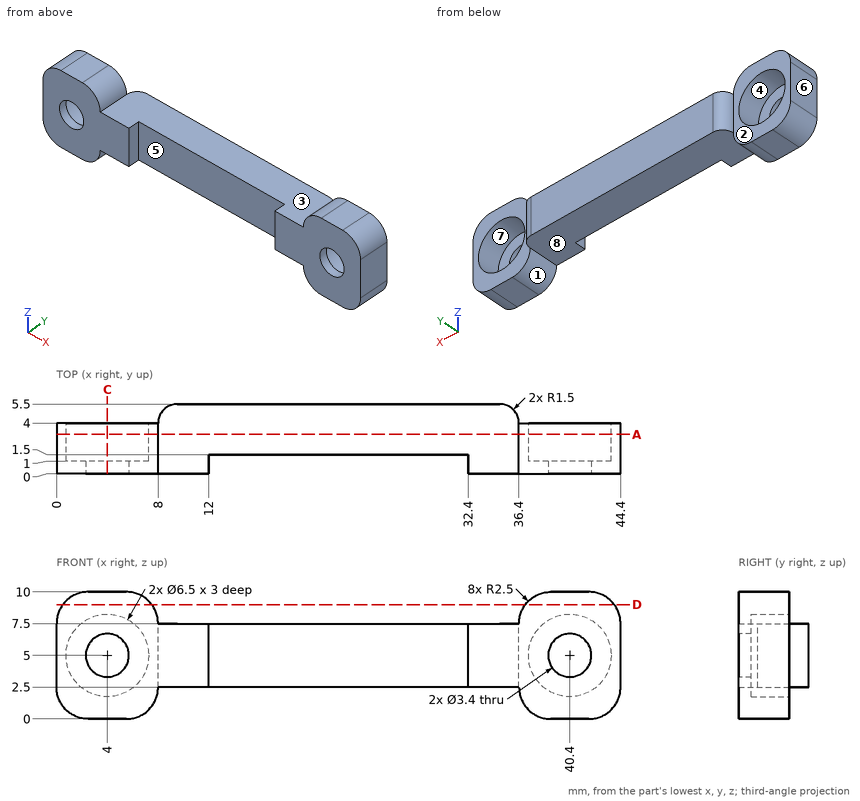
Job drawing, mm, ordinate dimensions from the low corner. One solid piece. A direction names the side the tool comes from. Give positions to 0.01 mm unless a question says otherwise; leave off trailing zeros. Order: outer loops, then holes, each group sorted by start corner. A loop starts at its lowest first (then second) coordinate and runs counter-clockwise, first axis right, second up. Notation, with made-up numbers: (-22, -26.75) -> (-11, -26.75) arc R31 cw to (-11, 5.25) -> close; hole circle Ø5 at (-33.5, 15). An arc over 180 degrees is marked (long way). Return JSON: item names as keys, results as strings.
Q1. Saw through at C-C (x = 4). Write the cut outline in (y, z), then the cut area to 3 significant figures.
Working result:
{"outline": "(0, 0) -> (4, 0) -> (4, 1.75) -> (1, 1.75) -> (1, 3.3) -> (0, 3.3) -> close; (0, 6.7) -> (1, 6.7) -> (1, 8.25) -> (4, 8.25) -> (4, 10) -> (0, 10) -> close", "area": "17.1 mm²"}
Q2. Saw through at A-A (y = 3.1). Count the separate pieces of the cut face and the enclosed holes in it, then the cut area to 3 significant figures.
Working result:
{"separate pieces": "1", "enclosed holes": "2", "area": "225 mm²"}
Q3. Mould opens along Z. For the marked faces 6, 7 and 8 say: pulls with the +Z half, pulls with the -Z half, needs draft (parallel to the pull), parting line crosses it, or undercut.
Working result:
{"face 6": "needs draft", "face 7": "undercut", "face 8": "pulls with the -Z half"}
Q4. Which spindle directions (+Z, -Z, +X, -X, +Y, -Y) get a long thin tool onto all of the face, cutting with end or side? Do the marked faces 1, 2, 3, 4 and 5. Say none if no direction does.
Working result:
{"face 1": "-Z, +Y, -Y", "face 2": "+Z, -Z, -X, +Y", "face 3": "+Z, +Y, -Y", "face 4": "+Y", "face 5": "+Z, -Z, -Y"}
Q5. Drill centre lines: line 1 (X direction, y = 0.75, z = 5); line 2 (X direction, y = 1.7, z = 4.75); line 3 (Z direction, x = 4, y = 2.05). Where is each one in solid material? Low to high.
Working result:
{"line 1": "0 to 2.3, 5.7 to 12, 32.4 to 38.7, 42.1 to 44.4", "line 2": "0 to 0.76, 7.24 to 37.16, 43.64 to 44.4", "line 3": "0 to 1.75, 8.25 to 10"}
Q6. Flat gauge pins, fed straight in: pin 1 (2.5 mm diameter, centred on x = 39.5, z = 6.5, fed in from +Y); pin 2 (1.5 mm diameter, centred on x = 34.5, y = 2, fed in from +Z); pin 3 (3 mm diameter, centred on x = 29, y = 4, fed in from -Z). Where does each tip first touch, or does it go through?
Working result:
{"pin 1": "y = 1", "pin 2": "z = 7.5", "pin 3": "z = 2.5"}
Q7. Saw through at D-D (z = 9). Write the cut outline in (x, y), then the cut area to 3 significant figures.
Working result:
{"outline": "(0.5, 0) -> (7.5, 0) -> (7.5, 4) -> (0.5, 4) -> close; (36.9, 0) -> (43.9, 0) -> (43.9, 4) -> (36.9, 4) -> close", "area": "56.0 mm²"}
